```python
from build123d import *

# Parameters (mm, degrees)
SKETCH_1_W                     = 10
SKETCH_1_H                     = 6
EXTRUDE_1_DEPTH                = 1
SKETCH_2_W                     = 1
SKETCH_2_H                     = 6
EXTRUDE_2_DEPTH                = 10
HOLE_WIZARD_M1_6_2_D           = 1.25
HOLE_WIZARD_M1_6_2_CSINK_D     = 1.65
HOLE_WIZARD_M1_6_2_CSINK_ANGLE = 90
HOLE_WIZARD_M1_6_4_D           = 1.25
HOLE_WIZARD_M1_6_4_CSINK_D     = 1.65
HOLE_WIZARD_M1_6_4_CSINK_ANGLE = 90


# Read off the part's stored shape, not the designer's step: M1.6 螺纹孔3
with BuildPart() as part:
    # 草图1 → 凸台-拉伸1 (new body)
    with BuildSketch(Plane(origin=(0, 0, 0), x_dir=(1, 0, 0), z_dir=(0, 1, 0))):
        Rectangle(SKETCH_1_W, SKETCH_1_H)
    extrude(amount=EXTRUDE_1_DEPTH)

    # 草图2 → 凸台-拉伸2 (add)
    with BuildSketch(Plane(origin=(0, 1, 0), x_dir=(1, 0, 0), z_dir=(0, 1, 0))):
        with Locations((-4.5, 0)):
            Rectangle(SKETCH_2_W, SKETCH_2_H)
    extrude(amount=EXTRUDE_2_DEPTH)

    # M1.6 螺纹孔2 (through all)
    with Locations(Plane(origin=(-4, 0, 0), x_dir=(0, 0, -1), z_dir=(1, 0, 0))):
        with Locations((-1.8, 9.7), (1.8, 9.7)):
            CounterSinkHole(HOLE_WIZARD_M1_6_2_D / 2, HOLE_WIZARD_M1_6_2_CSINK_D / 2, counter_sink_angle=HOLE_WIZARD_M1_6_2_CSINK_ANGLE)

    # M1.6 螺纹孔3 outline → M1.6 螺纹孔3 (revolve, cut)
    with BuildSketch(Plane(origin=(3.8, 0, 1.8), x_dir=(1, 0, 0), z_dir=(0, 0, 1))):
        Polygon((0, 0), (0.625, 0), (0.625, 0.8), (0.825, 1), (0, 1), align=None)
    revolve(axis=Axis((3.8, 0, 1.8), (0, 1, 0)), mode=Mode.SUBTRACT)

    # Hole Wizard M1.6 _3 2 outline → Hole Wizard M1.6 _3 2 (revolve, cut)
    with BuildSketch(Plane(origin=(3.8, 0, -1.8), x_dir=(1, 0, 0), z_dir=(0, 0, 1))):
        Polygon((0, 0), (0.625, 0), (0.625, 0.8), (0.825, 1), (0, 1), align=None)
    revolve(axis=Axis((3.8, 0, -1.8), (0, 1, 0)), mode=Mode.SUBTRACT)

    # M1.6 螺纹孔4 (through all)
    with Locations(Plane(origin=(0, 1, 0), x_dir=(1, 0, 0), z_dir=(0, 1, 0))):
        with Locations((-2.2, -1.8), (-2.2, 1.8)):
            CounterSinkHole(HOLE_WIZARD_M1_6_4_D / 2, HOLE_WIZARD_M1_6_4_CSINK_D / 2, counter_sink_angle=HOLE_WIZARD_M1_6_4_CSINK_ANGLE)


solid = part.part
```
Input: part model. Units: mm. Frame: model coordinates. Coordinates: 2 decimals unless noted, no trailing zeros. Write each loop counter-clockwise with the first axis right and the second up, starting at its lowest first coordinate (ties: lowest second). Pieces come first, ordered by that corner, then holes.
1) Section C-C on y = 9.7. Output: boundary loops of the cut face in (x, z) (3 decimals), and give its area (3 significant figures).
2) Section B-B on z = 1.8. Output: boundary loops of the cut face in (x, y) (3 decimals).
3) Material intervals for line 1 along Z through (x, y) = (-2.2, 0.4) (3 decimals); line 2 along Y through (x, z) = (-4.6, -1.8) (3 decimals); line 3 along X through (y, z) = (0.75, -1.65), sorted ascending.
4) Section A-A on x = -2.2. Output: boundary loops of the cut face in (y, z) (3 decimals), and give its area (3 significant figures).
5) Section D-D on z = 0.8. Output: boundary loops of the cut face in (x, y), and give its area (3 significant figures).
6) Pin query (flat end, axial travel): pin 1 Ø3 at (y, z) = (7, 1) entering from +X; pin 2 Ø3 at (x, z) = (2, -1) entering from +Y. Return the tip coordinate at first contact, or that it passes through.
7) Mould query, pull axis X, two halves, no side actions, for faces 1 (the cylindrical face through (3.72, 0.41, 1.18)), 2 (the cylindrical face through (-4.61, 9.09, 1.66)), 3 (the flat face through (-4, 6, 0)). Classes: pulls with the +X half, pulls with the -X half, needs draft (parallel to the pull), parting line crosses it, or undercut.
Check result:
1. outline: (-5, -3) - (-4, -3) - (-4, -2.625) - (-4.2, -2.425) - (-5, -2.425) - close; (-5, -1.175) - (-4.2, -1.175) - (-4, -0.975) - (-4, 0.975) - (-4.2, 1.175) - (-5, 1.175) - close; (-5, 2.425) - (-4.2, 2.425) - (-4, 2.625) - (-4, 3) - (-5, 3) - close
1. area: 3.42 mm2
2. outline: (-5, 0) - (-2.825, 0) - (-2.825, 0.8) - (-3.025, 1) - (-4, 1) - (-4, 8.875) - (-4.2, 9.075) - (-5, 9.075) - close; (-5, 10.325) - (-4.2, 10.325) - (-4, 10.525) - (-4, 11) - (-5, 11) - close; (-1.575, 0) - (3.175, 0) - (3.175, 0.8) - (2.975, 1) - (-1.375, 1) - (-1.575, 0.8) - close; (4.425, 0) - (5, 0) - (5, 1) - (4.625, 1) - (4.425, 0.8) - close
3. line 1: z = -3 to -2.425, -1.175 to 1.175, 2.425 to 3
3. line 2: y = 0 to 9.075, 10.325 to 11
3. line 3: x = -5 to -2.81, -1.59 to 3.19, 4.41 to 5
4. outline: (0, -3) - (1, -3) - (1, -2.625) - (0.8, -2.425) - (0, -2.425) - close; (0, -1.175) - (0.8, -1.175) - (1, -0.975) - (1, 0.975) - (0.8, 1.175) - (0, 1.175) - close; (0, 2.425) - (0.8, 2.425) - (1, 2.625) - (1, 3) - (0, 3) - close
4. area: 3.42 mm2
5. outline: (-5, 0) - (5, 0) - (5, 1) - (-4, 1) - (-4, 11) - (-5, 11) - close
5. area: 20.0 mm2
6. pin 1: stops at x = -4
6. pin 2: stops at y = 1
7. face 1: undercut
7. face 2: needs draft
7. face 3: pulls with the +X half
